Geometry: see drawing. Coordinates: mm, zero at the bounding-box minimum. A direction names the side the tool comes from. Give positions to 0.01 mm unless a question says otherwise; leave off trailing zeros. Loops run counter-clockwise (first coordinate to the right, second up) from the corner with the lowest first, then second, coordinate; pieces in that order, holes last. Notation, with made-up numbers: (-27.75, -12.5) - (-4.75, -12.5) arc R10 ccw to (-4.75, 2.5) - close; hole circle Ø2 at (35, -1.75). An arc over 180 degrees is marked (long way). Use CSV: the item, a comma, the result in double quotes. Start each with the question number.
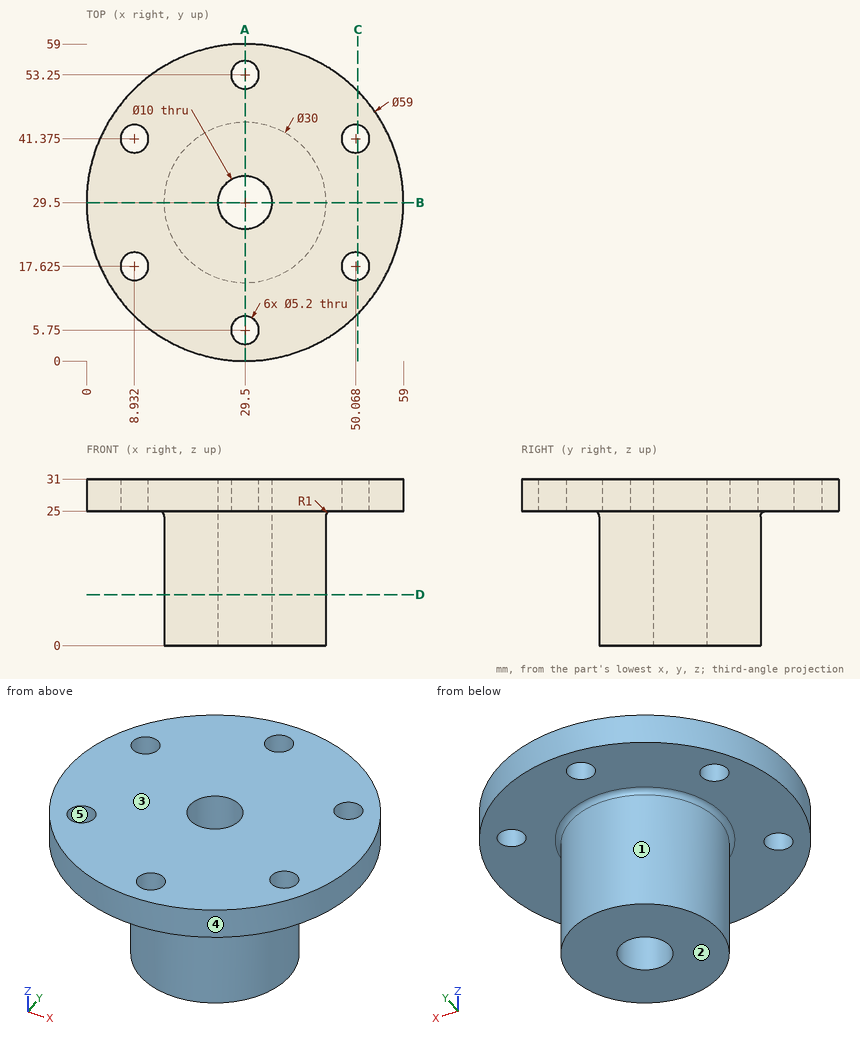
Item 1: Reachability of the marked faces 1 and 2 from +Z, -Z, +X, -X, +Y, -Y: full face, straight path, thin tool, end or side. Return the list, or none.
Item 2: Section C-C (x = 50.5). Output: boundary loops of the cut face in (y, z).
Item 3: Section A-A (x = 29.5). Output: boundary loops of the cut face in (y, z), plus the area to 3 significant figures.
Item 4: Mould query, pull axis Y, two halves, no side actions, for the marked faces 3, 4 and 5. Classes: pulls with the +Y half, pulls with the -Y half, needs draft (parallel to the pull), parting line crosses it, or undercut.
Item 5: Pin query (flat end, axial travel): pin 1 Ø4.5 at (x, y) = (8.93, 41.38) entering from -Z; pin 2 Ø12 at (y, z) = (47.5, 6) entering from -X; pin 3 Ø5 at (x, z) = (32, 23.5) entering from -Y; pin 4 Ø6 at (y, z) = (30.5, 15.5) entering from +X. Return the tip coordinate at first contact, or that it passes through.
Item 6: Section B-B (y = 29.5). Output: boundary loops of the cut face in (x, z), plus the area to 3 significant figures.
Item 7: Ray query, probe 1 along Z at (x, y) = (42.5, 13); probe 2 along Y at (x, z) = (27, 13); probe 3 along Y at (x, z) = (29.5, 19.5). Return the intervals inside material, ascending.
Item 8: Section D-D (z = 9.5). Output: boundary loops of the cut face in (x, y), plus the area to 3 significant figures.
Outcome:
1,face 1,"-Z"
1,face 2,"-Z, +X, -X, +Y, -Y"
2,outline,"(8.78, 25) - (15.06, 25) - (15.06, 31) - (8.78, 31) - close; (20.19, 25) - (38.81, 25) - (38.81, 31) - (20.19, 31) - close; (43.94, 25) - (50.22, 25) - (50.22, 31) - (43.94, 31) - close"
3,outline,"(0, 25) - (3.15, 25) - (3.15, 31) - (0, 31) - close; (8.35, 25) - (13.5, 25) arc R1 cw to (14.5, 24) - (14.5, 0) - (24.5, 0) - (24.5, 31) - (8.35, 31) - close; (34.5, 0) - (44.5, 0) - (44.5, 24) arc R1 cw to (45.5, 25) - (50.65, 25) - (50.65, 31) - (34.5, 31) - close; (55.85, 25) - (59, 25) - (59, 31) - (55.85, 31) - close"
3,area,"732 mm2"
4,face 3,"needs draft"
4,face 4,"parting line crosses it"
4,face 5,"undercut"
5,pin 1,"passes through"
5,pin 2,"stops at x = 20.5"
5,pin 3,"stops at y = 0"
5,pin 4,"stops at x = 44.5"
6,outline,"(0, 25) - (13.5, 25) arc R1 cw to (14.5, 24) - (14.5, 0) - (24.5, 0) - (24.5, 31) - (0, 31) - close; (34.5, 0) - (44.5, 0) - (44.5, 24) arc R1 cw to (45.5, 25) - (59, 25) - (59, 31) - (34.5, 31) - close"
6,area,"794 mm2"
7,probe 1,"z = 25 to 31"
7,probe 2,"y = 14.71 to 25.17, 33.83 to 44.29"
7,probe 3,"y = 14.5 to 24.5, 34.5 to 44.5"
8,outline,"circle Ø30 at (29.5, 29.5); hole circle Ø10 at (29.5, 29.5)"
8,area,"628 mm2"
